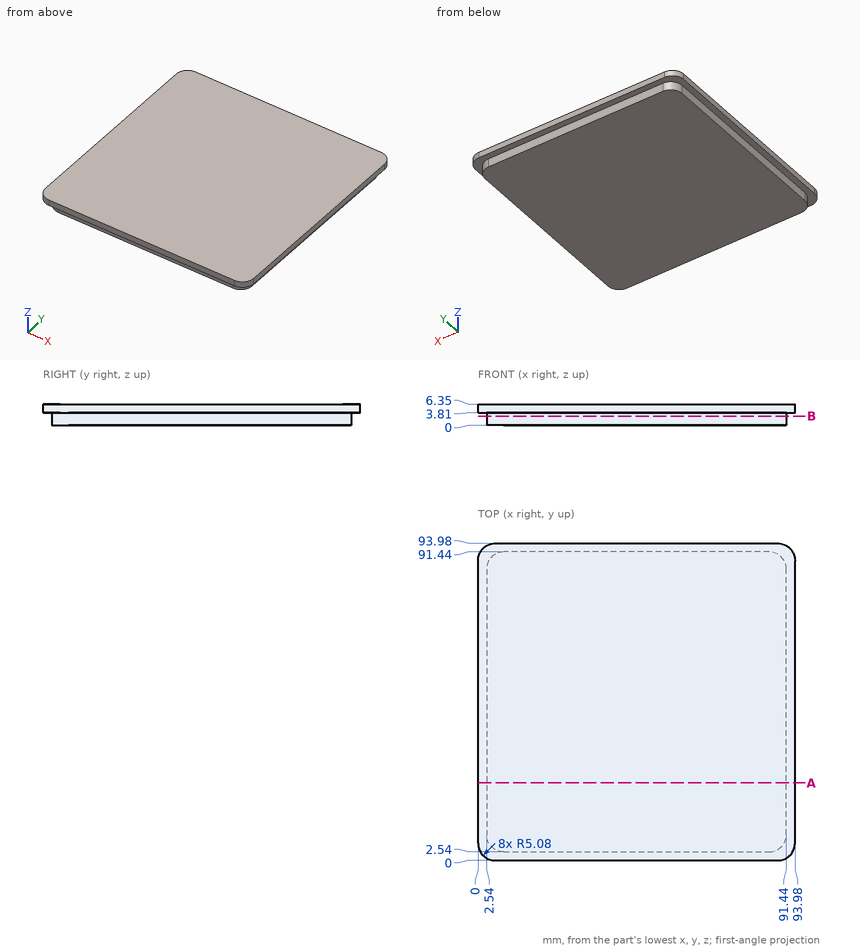
Source: three-view drawing plus pictorial views. Frame: mm from the lowest corner of the part. Coordinates: 2 decimals unless noted, no trailing zeros. Order: outer loops, then holes, each group sorted by start corner. A loop starts at its lowest first (then second) coordinate and runs counter-clockwise, first axis right, second up. Notation, with made-up numbers: M 23.5,28.25 L 32.5,28.25 A25 cw 32.5,52.25 Z; hole C 17.25,16 d4. An arc over 180 degrees is marked long. One line per question, with ' | ' between items.
Item 1: Pin query (flat end, axial travel): pin 1 (1.1 mm diameter, centred on x = 40.5, z = 1.5, fed in from -Y); pin 2 (1.1 mm diameter, centred on x = 49.5, z = 1.5, fed in from +Y); pin 3 (1.9 mm diameter, centred on y = 49, z = 1, fed in from -X). Return the tip coordinate at first contact, or that it passes through.
Geometry results:
pin 1: stops at y = 2.54 | pin 2: stops at y = 91.44 | pin 3: stops at x = 2.54
Item 2: Ray query, line 1 along Y through (x, z) = (23.5, 1.75); line 2 along Y through (x, z) = (88, 2.75). Return the intervals inside material, ascending.
Geometry results:
line 1: y = 2.54 to 91.44 | line 2: y = 2.81 to 91.17
Item 3: Section B-B (z = 2.75). Output: boundary loops of the cut face in (x, y), then the cut area to 3 significant figures.
Geometry results:
outline: M 2.54,7.62 A5.08 ccw 7.62,2.54 L 86.36,2.54 A5.08 ccw 91.44,7.62 L 91.44,86.36 A5.08 ccw 86.36,91.44 L 7.62,91.44 A5.08 ccw 2.54,86.36 Z | area: 7,880 mm^2
Item 4: Section A-A (y = 23). Output: boundary loops of the cut face in (x, z), then the cut area to 3 significant figures.
Geometry results:
outline: M 0,3.81 L 2.54,3.81 L 2.54,0 L 91.44,0 L 91.44,3.81 L 93.98,3.81 L 93.98,6.35 L 0,6.35 Z | area: 577 mm^2
